```python
from build123d import *

# Parameters (mm, degrees)
F0_R     = 12.5
F1_DEPTH = 7
F2_W     = 13.25
F2_H     = 13.25
F2_W_2   = 9
F2_H_2   = 9
F2_H_3   = 13.5
F3_DEPTH = 1
F4_DEPTH = 5


with BuildPart() as f1:
    # F0 (on Top) → F1 (new body)
    with BuildSketch(Plane.XY):
        with BuildLine():
            ThreePointArc((0, 17.5), (5.125631, 5.125631), (17.5, 0))
            Line((17.5, 0), (85, 0))
            ThreePointArc((85, 0), (88.535534, 1.464466), (90, 5))
            Line((90, 5), (90, 30))
            ThreePointArc((90, 30), (88.535534, 33.535534), (85, 35))
            Line((85, 35), (17.5, 35))
            ThreePointArc((17.5, 35), (5.125631, 29.874369), (0, 17.5))
        make_face()
        with Locations((17.5, 17.5)):
            Circle(F0_R, mode=Mode.SUBTRACT)
    extrude(amount=F1_DEPTH)

    # F2 (on face) → F3 (join)
    with BuildSketch(Plane.XY.offset(7)):
        with Locations((41.625, 26.375)):
            Rectangle(F2_W, F2_H)
        with Locations((41.625, 26.375)):
            Rectangle(F2_W_2, F2_H_2, mode=Mode.SUBTRACT)
        with Locations((41.625, 8.75)):
            Rectangle(F2_W, F2_H_3)
        with Locations((41.625, 8.75)):
            Rectangle(F2_W_2, F2_H_2, mode=Mode.SUBTRACT)
        with Locations((59.875, 17.5)):
            Rectangle(F2_W, F2_H)
        with Locations((59.875, 17.5)):
            Rectangle(F2_W_2, F2_H_2, mode=Mode.SUBTRACT)
        with Locations((78.125, 8.625)):
            Rectangle(F2_W, F2_H)
        with Locations((78.125, 8.625)):
            Rectangle(F2_W_2, F2_H_2, mode=Mode.SUBTRACT)
        with Locations((78.125, 26.375)):
            Rectangle(F2_W, F2_H)
        with Locations((78.125, 26.375)):
            Rectangle(F2_W_2, F2_H_2, mode=Mode.SUBTRACT)
    extrude(amount=F3_DEPTH)

    # F2 (on face) → F4 (cut)
    with BuildSketch(Plane.XY.offset(7)):
        with Locations((41.625, 26.375)):
            Rectangle(F2_W_2, F2_H_2)
        with Locations((41.625, 8.75)):
            Rectangle(F2_W_2, F2_H_2)
        with Locations((59.875, 17.5)):
            Rectangle(F2_W_2, F2_H_2)
        with Locations((78.125, 26.375)):
            Rectangle(F2_W_2, F2_H_2)
        with Locations((78.125, 8.625)):
            Rectangle(F2_W_2, F2_H_2)
    extrude(amount=-F4_DEPTH, mode=Mode.SUBTRACT)


solid = f1.part
```
The model under review builds one solid part; all positions refer to its coordinate system, in mm. A direction names the side the tool comes from. Coordinates: 2 decimals unless noted, no trailing zeros. Write each loop counter-clockwise with the first axis right and the second up, starting at its lowest first coordinate (ties: lowest second). Pieces come first, ordered by that corner, then holes.
1) Clearance check with flat-ended pins moving along their axes: pin 1 Ø7 at (x, y) = (42, 8) entering from +Z; pin 2 Ø0.8 at (x, z) = (75.5, 7.5) entering from -Y; pin 3 Ø0.5 at (x, z) = (78.5, 7.5) entering from +Y. State where each tip first meets the part, or that it passes through.
2) We need section A-A on x = 40. State the section outline as (y, z) points (3 decimals).
3) We need section B-B on x = 13. State the section outline as (y, z) points, then the cut area to 3 significant figures.
4) To check wall thickness, follow probe 1 along X at (y, z) = (7.5, 5) (3 decimals); probe 2 along X at (y, z) = (30.5, 5.5) (3 decimals); probe 3 along X at (y, z) = (12, 6) (3 decimals). State the ranges of each line that lie inside material, in increasing order.
5) The part is to be moulded in two halves that separate along Y. For faces 3 (the face through (90, 17, 3)), 4 (the face through (52, 35, 3)), 5 (the face through (64.375, 17, 5)), 6 (the face through (78, 26, 2)), say which applies: pulls with the +Y half, pulls with the -Y half, needs draft (parallel to the pull), parting line crosses it, or undercut.
6) Machinability: for faces 1 (the face through (14.79, 5.297, 3.451)), 2 (the face through (60, 22, 5)), which of the approach directions +Z, -Z, +X, -X, +Y, -Y give a long, thin tool a straight path to every point of the face, cutting with its end or side? Answer none if there is none.
Answer list:
1. pin 1: stops at z = 2
1. pin 2: stops at y = 2
1. pin 3: stops at y = 33
2. outline: (0, 0) - (35, 0) - (35, 7) - (33, 7) - (33, 8) - (30.875, 8) - (30.875, 2) - (21.875, 2) - (21.875, 8) - (19.75, 8) - (19.75, 7) - (15.5, 7) - (15.5, 8) - (13.25, 8) - (13.25, 2) - (4.25, 2) - (4.25, 8) - (2, 8) - (2, 7) - (0, 7) - close
3. outline: (0.59, 0) - (5.84, 0) - (5.84, 7) - (0.59, 7) - close; (29.16, 0) - (34.41, 0) - (34.41, 7) - (29.16, 7) - close
3. area: 73.5 mm2
4. probe 1: x = 3.139 to 10, 25 to 37.125, 46.125 to 73.625, 82.625 to 90
4. probe 2: x = 5.785 to 37.125, 46.125 to 73.625, 82.625 to 89.975
4. probe 3: x = 0.887 to 6.275, 28.725 to 37.125, 46.125 to 73.625, 82.625 to 90
5. face 3: needs draft
5. face 4: pulls with the +Y half
5. face 5: undercut
5. face 6: undercut
6. face 1: +Z, -Z
6. face 2: +Z
